Input: part model. Units: mm. Frame: model coordinates. A direction names the side the tool comes from. Give positions to 0.01 mm unless a question says otherwise; leave off trailing zeros. Loops run counter-clockwise (first coordinate to the right, second up) from the corner with the lowest first, then second, coordinate; pieces in that order, holes last. Notation, with made-up numbers: (24.25, 21) -> (61.25, 21) arc R5 cw to (61.25, 25) -> close; hole circle Ø1 at (45.5, 26). An arc over 180 degrees is marked (long way). One line per question, with ' | ' between items.
from build123d import *

# Parameters (mm, degrees)
F0_W     = 76.2
F0_H     = 76.2
F1_DEPTH = 76.2
F2_T     = -3.175
F3_R     = 5.08


with BuildPart() as f1:
    # F0 (on Front) → F1 (new body)
    with BuildSketch(Plane.XZ):
        with Locations((7.068123761, -2.0512547344)):
            Rectangle(F0_W, F0_H)
    extrude(amount=F1_DEPTH)

    # F2
    f2_openings = [f1.faces().sort_by_distance(p)[0] for p in [
        (7.068124, -76.2, -2.051255),
        (7.068124, 0, -2.051255),
    ]]
    offset(amount=F2_T, openings=f2_openings)

    # F3
    f3_edges = [f1.edges().sort_by_distance(p)[0] for p in [
        (-27.856876, -38.1, 32.873745),
        (41.993124, -38.1, -36.976255),
        (41.993124, -38.1, 32.873745),
        (-31.031876, -38.1, -40.151255),
        (45.168124, -38.1, -40.151255),
        (45.168124, -38.1, 36.048745),
        (-31.031876, -38.1, 36.048745),
        (-27.856876, -38.1, -36.976255),
    ]]
    fillet(f3_edges, radius=F3_R)


solid = f1.part
1. Section query B-B (z = -15.5). Output: boundary loops of the cut face in (x, y).
Determined:
outline: (-31.03, -76.2) -> (-27.86, -76.2) -> (-27.86, 0) -> (-31.03, 0) -> close; (41.99, -76.2) -> (45.17, -76.2) -> (45.17, 0) -> (41.99, 0) -> close
2. Reachability of faces 5 (the flat face through (7, -38, 32.874)), 6 (the cylindrical face through (43.72, -38.63, 34.52)) from +Z, -Z, +X, -X, +Y, -Y: full face, straight path, thin tool, end or side. Return the list, or none.
Determined:
face 5: +Y, -Y | face 6: +Z, +X, +Y, -Y
3. Section query A-A (x = 34.5). Output: boundary loops of the cut face in (y, z).
Determined:
outline: (-76.2, -40.15) -> (0, -40.15) -> (0, -36.98) -> (-76.2, -36.98) -> close; (-76.2, 32.87) -> (0, 32.87) -> (0, 36.05) -> (-76.2, 36.05) -> close
4. Ray query, line 1 along Z through (x, y) = (-15, -27); line 2 along X through (y, z) = (-63, 3.5); line 3 along X through (y, z) = (-13.5, 29). Return the intervals inside material, ascending. Write a range as from..to.
Determined:
line 1: z = -40.15..-36.98, 32.87..36.05 | line 2: x = -31.03..-27.86, 41.99..45.17 | line 3: x = -31.03..-27.71, 41.85..45.17
5. Pull-direction query (X, two-part tool) for faces 1 (the flat face through (7, -38, 36.049)), 2 (the cylindrical face through (-26.408, -37.567, -35.449)), 3 (the flat face through (7, -38, -36.976)), 4 (the flat face through (-31.032, -38, -3)); classes: pulls with the +X half, pulls with the -X half, needs draft (parallel to the pull), parting line crosses it, or undercut.
Determined:
face 1: needs draft | face 2: undercut | face 3: undercut | face 4: pulls with the -X half
6. Section query C-C (y = -64.5). Output: boundary loops of the cut face in (x, z).
Determined:
outline: (-31.03, -35.07) arc R5.08 ccw to (-25.95, -40.15) -> (40.09, -40.15) arc R5.08 ccw to (45.17, -35.07) -> (45.17, 30.97) arc R5.08 ccw to (40.09, 36.05) -> (-25.95, 36.05) arc R5.08 ccw to (-31.03, 30.97) -> close; hole (-27.86, -31.9) arc R5.08 ccw to (-22.78, -36.98) -> (36.91, -36.98) arc R5.08 ccw to (41.99, -31.9) -> (41.99, 27.79) arc R5.08 ccw to (36.91, 32.87) -> (-22.78, 32.87) arc R5.08 ccw to (-27.86, 27.79) -> close
